```python
from build123d import *

# Parameters (mm, degrees)
BOSS_EXTRUDE1_DEPTH = 7
CIRPATTERN1_COUNT   = 11
CUT_EXTRUDE1_DEPTH  = 5
SKETCH4_R           = 11.25
SKETCH4_R_2         = 4
CUT_EXTRUDE2_DEPTH  = 2.5
CUT_EXTRUDE3_START  = -1
SKETCH6_R           = 11.25
CUT_EXTRUDE3_DEPTH  = 1
CHAMFER1_SIZE       = 0.5
FILLET1_R           = 0.25
FILLET2_R           = 0.2
CHAMFER2_SIZE       = 0.5
CHAMFER2_SIZE_2     = 1.866025404


with BuildPart() as part:
    # Sketch1 → Revolve1 (revolve)
    with BuildSketch(Plane(origin=(0, 0, 0), x_dir=(0, 0, -1), z_dir=(1, 0, 0)), mode=Mode.PRIVATE) as revolve1_sk:
        Polygon((0, 12.7), (7, 12.7), (7, 11.7), (6.5, 11.7), (6.5, 0), (0, 0), align=None)
    revolve(revolve1_sk.sketch.rotate(Axis((0, 0, 9.434023018), (0, 0, -1)), 90), axis=Axis((0, 0, 9.434023018), (0, 0, -1)))

    # Sketch2 → Boss-Extrude1 (add)
    with BuildSketch(Plane.XY):
        with BuildLine():
            Line((-0.75, 12.677834989), (-0.75, 13.2))
            ThreePointArc((-0.75, 13.2), (0, 13.95), (0.75, 13.2))
            Line((0.75, 13.2), (0.75, 12.677834989))
            ThreePointArc((0.75, 12.677834989), (0, 11.927834989), (-0.75, 12.677834989))
        make_face()
    boss_extrude1 = extrude(amount=-BOSS_EXTRUDE1_DEPTH)

    # CirPattern1: Boss-Extrude1 ×11 about axis
    cirpattern1_axis = Axis((0, 0, 0), (0, 0, 1))
    for i in range(1, CIRPATTERN1_COUNT):
        add(boss_extrude1.rotate(cirpattern1_axis, i * 360 / CIRPATTERN1_COUNT))

    # Sketch3 → Cut-Extrude1 (cut)
    with BuildSketch(Plane.XY):
        with BuildLine():
            Line((-0.95, 2.332380758), (-0.95, 1.45))
            ThreePointArc((-0.95, 1.45), (-1.096446609, 1.096446609), (-1.45, 0.95))
            Line((-1.45, 0.95), (-2.332380758, 0.95))
            ThreePointArc((-2.332380758, 0.95), (-2.457737974, 0.507737974), (-2.5, 0.05))
            Line((-2.5, 0.05), (-2.5, -0.05))
            ThreePointArc((-2.5, -0.05), (-2.457737974, -0.507737974), (-2.332380758, -0.95))
            Line((-2.332380758, -0.95), (-1.45, -0.95))
            ThreePointArc((-1.45, -0.95), (-1.096446609, -1.096446609), (-0.95, -1.45))
            Line((-0.95, -1.45), (-0.95, -2.332380758))
            ThreePointArc((-0.95, -2.332380758), (-0.507737974, -2.457737974), (-0.05, -2.5))
            Line((-0.05, -2.5), (0.05, -2.5))
            ThreePointArc((0.05, -2.5), (0.507737974, -2.457737974), (0.95, -2.332380758))
            Line((0.95, -2.332380758), (0.95, -1.45))
            ThreePointArc((0.95, -1.45), (1.096446609, -1.096446609), (1.45, -0.95))
            Line((1.45, -0.95), (2.332380758, -0.95))
            ThreePointArc((2.332380758, -0.95), (2.457737974, -0.507737974), (2.5, -0.05))
            Line((2.5, -0.05), (2.5, 0.05))
            ThreePointArc((2.5, 0.05), (2.457737974, 0.507737974), (2.332380758, 0.95))
            Line((2.332380758, 0.95), (1.45, 0.95))
            ThreePointArc((1.45, 0.95), (1.096446609, 1.096446609), (0.95, 1.45))
            Line((0.95, 1.45), (0.95, 2.332380758))
            ThreePointArc((0.95, 2.332380758), (0.507737974, 2.457737974), (0.05, 2.5))
            Line((0.05, 2.5), (-0.05, 2.5))
            ThreePointArc((-0.05, 2.5), (-0.507737974, 2.457737974), (-0.95, 2.332380758))
        make_face()
    extrude(amount=-CUT_EXTRUDE1_DEPTH, mode=Mode.SUBTRACT)

    # Sketch4 → Cut-Extrude2 (cut)
    with BuildSketch(Plane.XY):
        Circle(SKETCH4_R)
        Circle(SKETCH4_R_2, mode=Mode.SUBTRACT)
    extrude(amount=-CUT_EXTRUDE2_DEPTH, mode=Mode.SUBTRACT)

    # Sketch6 → Cut-Extrude3 (cut)
    with BuildSketch(Plane.XY.offset(CUT_EXTRUDE3_START)):
        with BuildLine():
            Line((-6.223214922, 11.070754086), (-6.505518641, 11.510027246))
            ThreePointArc((-6.505518641, 11.510027246), (-7.541939404, 11.735486783), (-7.76739894, 10.69906602))
            Line((-7.76739894, 10.69906602), (-7.485095221, 10.25979286))
            ThreePointArc((-7.485095221, 10.25979286), (-9.598019594, 8.316731321), (-11.220603078, 5.948786983))
            Line((-11.220603078, 5.948786983), (-11.695581079, 6.165702168))
            ThreePointArc((-11.695581079, 6.165702168), (-12.689366335, 5.795039431), (-12.318703598, 4.801254175))
            Line((-12.318703598, 4.801254175), (-11.843725597, 4.58433899))
            ThreePointArc((-11.843725597, 4.58433899), (-12.570732312, 1.807398446), (-12.655529037, -1.061877955))
            Line((-12.655529037, -1.061877955), (-13.172379162, -1.136189784))
            ThreePointArc((-13.172379162, -1.136189784), (-13.808009114, -1.985291994), (-12.958906904, -2.620921947))
            Line((-12.958906904, -2.620921947), (-12.44205678, -2.546610117))
            ThreePointArc((-12.44205678, -2.546610117), (-11.552326341, -5.275770665), (-10.072413947, -7.735404145))
            Line((-10.072413947, -7.735404145), (-10.467039932, -8.077349507))
            ThreePointArc((-10.467039932, -8.077349507), (-10.542706562, -9.135307239), (-9.484748831, -9.210973869))
            Line((-9.484748831, -9.210973869), (-9.090122846, -8.869028506))
            ThreePointArc((-9.090122846, -8.869028506), (-6.866138382, -10.683919867), (-4.291378597, -11.952994175))
            Line((-4.291378597, -11.952994175), (-4.438489481, -12.454007834))
            ThreePointArc((-4.438489481, -12.454007834), (-3.930169168, -13.384926982), (-2.99925002, -12.876606669))
            Line((-2.99925002, -12.876606669), (-2.852139136, -12.37559301))
            ThreePointArc((-2.852139136, -12.37559301), (0, -12.7), (2.852139136, -12.37559301))
            Line((2.852139136, -12.37559301), (2.99925002, -12.876606669))
            ThreePointArc((2.99925002, -12.876606669), (3.930169168, -13.384926982), (4.438489481, -12.454007834))
            Line((4.438489481, -12.454007834), (4.291378597, -11.952994175))
            ThreePointArc((4.291378597, -11.952994175), (6.866138382, -10.683919867), (9.090122846, -8.869028506))
            Line((9.090122846, -8.869028506), (9.484748831, -9.210973869))
            ThreePointArc((9.484748831, -9.210973869), (10.542706562, -9.135307239), (10.467039932, -8.077349507))
            Line((10.467039932, -8.077349507), (10.072413947, -7.735404145))
            ThreePointArc((10.072413947, -7.735404145), (11.552326341, -5.275770665), (12.44205678, -2.546610117))
            Line((12.44205678, -2.546610117), (12.958906904, -2.620921947))
            ThreePointArc((12.958906904, -2.620921947), (13.808009114, -1.985291994), (13.172379162, -1.136189784))
            Line((13.172379162, -1.136189784), (12.655529037, -1.061877955))
            ThreePointArc((12.655529037, -1.061877955), (12.570732312, 1.807398446), (11.843725597, 4.58433899))
            Line((11.843725597, 4.58433899), (12.318703598, 4.801254175))
            ThreePointArc((12.318703598, 4.801254175), (12.689366335, 5.795039431), (11.695581079, 6.165702168))
            Line((11.695581079, 6.165702168), (11.220603078, 5.948786983))
            ThreePointArc((11.220603078, 5.948786983), (9.598019594, 8.316731321), (7.485095221, 10.25979286))
            Line((7.485095221, 10.25979286), (7.76739894, 10.69906602))
            ThreePointArc((7.76739894, 10.69906602), (7.541939404, 11.735486783), (6.505518641, 11.510027246))
            Line((6.505518641, 11.510027246), (6.223214922, 11.070754086))
            ThreePointArc((6.223214922, 11.070754086), (3.578003472, 12.185560765), (0.75, 12.677834989))
            Line((0.75, 12.677834989), (0.75, 13.2))
            ThreePointArc((0.75, 13.2), (0, 13.95), (-0.75, 13.2))
            Line((-0.75, 13.2), (-0.75, 12.677834989))
            ThreePointArc((-0.75, 12.677834989), (-3.578003472, 12.185560765), (-6.223214922, 11.070754086))
        make_face()
        Circle(SKETCH6_R, mode=Mode.SUBTRACT)
    extrude(amount=CUT_EXTRUDE3_DEPTH, mode=Mode.SUBTRACT)

    # Chamfer1
    chamfer1_edges = [part.edges().sort_by_distance(p)[0] for p in [
        (-11.25, 0, -1),
    ]]
    chamfer(chamfer1_edges, length=CHAMFER1_SIZE)

    # Fillet1
    fillet1_edges = [part.edges().sort_by_distance(p)[0] for p in [
        (-11.25, 0, -2.5),
        (-4, 0, -2.5),
    ]]
    fillet(fillet1_edges, radius=FILLET1_R)

    # Fillet2
    fillet2_edges = [part.edges().sort_by_distance(p)[0] for p in [
        (-4, 0, 0),
    ]]
    fillet(fillet2_edges, radius=FILLET2_R)

    # Chamfer2
    # the kernel refuses this chamfer: 1.866025404, 0.5 mm, written as the material it adds along each edge
    with BuildSketch(Plane(origin=(0, 0, -6.5), x_dir=(1, 0, 0), z_dir=(0, 1, 0))) as chamfer2_piece_1_section:
        Polygon((11.7, CHAMFER2_SIZE), (11.7 - CHAMFER2_SIZE_2, 0), (11.7, 0), align=None)
    chamfer2_piece_1 = revolve(axis=Axis((0, 0, -6.5), (0, 0, -1)), mode=Mode.PRIVATE)
    chamfer2_piece_1 = split(chamfer2_piece_1, bisect_by=Plane(origin=(-10.739750949, 0, -7), z_dir=(0, 0, 1)), keep=Keep.TOP, mode=Mode.PRIVATE)
    add(chamfer2_piece_1)


solid = part.part
```
Input: part model. Units: mm. Frame: model coordinates. A direction names the side the tool comes from. Coordinates: 2 decimals unless noted, no trailing zeros. Put each result on its own line as item: value.
1. Reachability of faces 1 (the face through (-7.556, 11.726, -3.958)), 2 (the face through (3.539, 12.197, -4.042)), 3 (the face through (2, 0.95, -2)) from +Z, -Z, +X, -X, +Y, -Y: full face, straight path, thin tool, end or side. Return the list, or none.
Report:
face 1: +Z, -Z
face 2: +Z, -Z, +Y
face 3: +Z
2. Draft query along Y for faces 4 (the face through (2.46, 0.5, -2.46)), 5 (the face through (0, -5, -2.5)), 6 (the face through (-3.617, 12.174, -4.042)), 7 (the face through (12, 3, -7)). Return one class per face: pulls with the +Y half, pulls with the -Y half, needs draft (parallel to the pull), parting line crosses it, or undercut.
Report:
face 4: undercut
face 5: undercut
face 6: pulls with the +Y half
face 7: needs draft
3. Contact query for flat-ended pins moving along their axis: pin 1 Ø4 at (y, z) = (4.5, -1.5) entering from +X; pin 2 Ø12 at (x, y) = (-10, 7.5) entering from +Z; pin 3 Ø0.7 at (x, z) = (2, -2) entering from +Y. Output: stop coordinate, or through.
Report:
pin 1: stops at x = 12.76
pin 2: stops at z = -1
pin 3: stops at y = 12.59
4. Line query: line 1 along Y through (x, z) = (0, -1.65); line 2 along X through (y, z) = (-9.25, -5); line 3 along Z through (x, y) = (-5, 7). Output: solid intervals per line, ascending.
Report:
line 1: y = -12.7 to -11.25, -4 to -2.5, 2.5 to 4, 11.25 to 13.95
line 2: x = -10.42 to -9.53, -8.7 to 8.7, 9.53 to 10.42
line 3: z = -6.5 to -2.5
